Check sheet for the modelled part. Datum: model origin and axes. Units: mm. A direction names the side the tool comes from. Give positions to 0.01 mm unless a question says otherwise; leave off trailing zeros. Loops run counter-clockwise (first coordinate to the right, second up) from the corner with the lowest first, then second, coordinate; pieces in that order, holes last. Notation, with made-up numbers: M 7.5,-7 L 27.5,-7 A14 cw 27.5,10 Z; hole C 81.25,3.25 d1. An arc over 180 degrees is marked long. Put each result on its own line as item: value. Start each with the question number.
```python
from build123d import *

# Parameters (mm, degrees)
F0_W         = 38
F0_H         = 14
F1_DEPTH     = 15
F2_R         = 4.8895
F3_DEPTH     = 15.001
F4_W         = 30.8590809897
F4_H         = 5.2
F5_DEPTH     = 5
F7_DEPTH     = 15.001
F8_W         = 13.0838444641
F8_H         = 13.9913465828
F9_DEPTH     = 8
F11_R        = 0.75
F12_DEPTH    = 15.001
F13_R        = 0.5
F14_T1_DEPTH = 9.498744071
F14_T3_DEPTH = 10.5
F14_T5_DEPTH = 20


# Not quite as in the source:
# - a fillet or chamfer that OpenCascade refuses, or shapes differently, is made with other operations: its cross-section is extruded or revolved along the edge and cut away or added


with BuildPart() as f1:
    # F0 (on Top) → F1 (new body)
    with BuildSketch(Plane.XY):
        with Locations((19, 7)):
            Rectangle(F0_W, F0_H)
    extrude(amount=F1_DEPTH)

    # F2 (on face) → F3 (cut, through all)
    with BuildSketch(Plane.XY.offset(15)):
        with Locations((3, 7)):
            Circle(F2_R)
    extrude(amount=-F3_DEPTH, mode=Mode.SUBTRACT)

    # F4 (on face) → F5 (cut)
    with BuildSketch(Plane(origin=(0, 0, 0), x_dir=(1, 0, 0), z_dir=(0, 0, -1))):
        with Locations((22.5704595052, -7)):
            Rectangle(F4_W, F4_H)
    extrude(amount=-F5_DEPTH, mode=Mode.SUBTRACT)

    # F6 (on face) → F7 (cut, through all)
    with BuildSketch(Plane.XY.offset(15)):
        with BuildLine():
            ThreePointArc((7.60725, 3.1564017591), (4.0503160688, 1.0926455874), (0, 1.8038475773))
            Line((0, 1.8038475773), (0, 0))
            Line((0, 0), (11.143, 0))
            Line((11.143, 0), (11.1420263596, 1.9376011727))
            ThreePointArc((11.1420263596, 1.9376011727), (9.7949393865, 3.7659627841), (7.60725, 3.1564017591))
        make_face()
        with BuildLine():
            ThreePointArc((0, 12.1961524227), (4.0503160688, 12.9073544126), (7.60725, 10.8435982409))
            ThreePointArc((7.60725, 10.8435982409), (9.7949393865, 10.2340372159), (11.1420263596, 12.0623988273))
            Line((11.1420263596, 12.0623988273), (11.1420263596, 14))
            Line((11.1420263596, 14), (0, 14))
            Line((0, 14), (0, 12.1961524227))
        make_face()
    extrude(amount=-F7_DEPTH, mode=Mode.SUBTRACT)

    # F8 (on face) → F9 (cut)
    with BuildSketch(Plane(origin=(0, 0, 0), x_dir=(1, 0, 0), z_dir=(0, 0, -1))):
        with Locations((4.6010777679, -6.9956732914)):
            Rectangle(F8_W, F8_H)
    extrude(amount=-F9_DEPTH, mode=Mode.SUBTRACT)

    # F11 (on face) → F12 (cut, through all)
    with BuildSketch(Plane.XY.offset(15)):
        with Locations((35, 7)):
            Circle(F11_R)
    extrude(amount=-F12_DEPTH, mode=Mode.SUBTRACT)

    # F13
    f13_edges = [f1.edges().sort_by_distance(p)[0] for p in [
        (0, 10.860986, 11.5),
        (0, 3.139014, 11.5),
    ]]
    fillet(f13_edges, radius=F13_R)

    # F14: fillet of radius 1 on 5 edges, made by hand

    # F14_s2 → F14_t1 (cut)
    with BuildSketch(Plane.XY.offset(8)):
        with BuildLine():
            ThreePointArc((11.1424977547, 0.9994975022), (11.4355685293, 0.2927155813), (12.1424976284, 0))
            Line((12.1424976284, 0), (11.143, 0))
            Line((11.143, 0), (11.1424977547, 0.9994975022))
        make_face()
    extrude(amount=F14_T1_DEPTH, mode=Mode.SUBTRACT)

    # F14_s4 → F14_t3 (cut)
    with BuildSketch(Plane.XY.offset(-2.5)):
        with BuildLine():
            ThreePointArc((11.143, 1), (11.4358932188, 0.2928932188), (12.143, 0))
            Line((12.143, 0), (11.143, 0))
            Line((11.143, 0), (11.143, 1))
        make_face()
    extrude(amount=F14_T3_DEPTH, mode=Mode.SUBTRACT)

    # F14_s6 → F14_t5 (cut)
    with BuildSketch(Plane.XY.offset(-2.5)):
        with BuildLine():
            ThreePointArc((37, 0), (37.7071067812, 0.2928932188), (38, 1))
            Line((38, 1), (38, 0))
            Line((38, 0), (37, 0))
        make_face()
        with BuildLine():
            ThreePointArc((11.1420263596, 13), (11.4349195784, 13.7071067812), (12.1420263596, 14))
            Line((12.1420263596, 14), (11.1420263596, 14))
            Line((11.1420263596, 14), (11.1420263596, 13))
        make_face()
        with BuildLine():
            ThreePointArc((38, 13), (37.7071067812, 13.7071067812), (37, 14))
            Line((37, 14), (38, 14))
            Line((38, 14), (38, 13))
        make_face()
    extrude(amount=F14_T5_DEPTH, mode=Mode.SUBTRACT)


solid = f1.part
```
Q1. Section check C-C, the plane x = 3. Record the cut outline in (y, z), then the cut area to 3 significant figures.
Q2. Thickness scan on line 1 along Y through (x, z) = (35, 8); line 2 along Y through (x, z) = (3, 13); line 3 along X through (y, z) = (10.75, 0.75). Record the ranges inside material, lowest first. Write a range as [from, to].
Q3. Section check B-B, the plane x = 35. Record the cut outline in (y, z).
Q4. Section check D-D, the plane z = 9.75. Record the cut outline in (x, y).
Q5. Access from +Z, -Z, +X, -X, +Y, -Y to the whole of each face (thin tool, end or side, straight path). Record for faces 1 (the face through (3.992, 12.917, 11.549)), 2 (the face through (11.143, 7, 6)), 3 (the face through (24, 4.4, 2)).
Q6. Section check A-A, the plane z = 1.5. Record the cut outline in (x, y).
Q7. Depth check by flat-ended pin: P1, Ø1, axis at y = 8.5, z = 13.5, coming from the -X side; P2, Ø6.5, axis at y = 7, z = 3, coming from the -X side; P3, Ø2, axis at x = 7.5, y = 9.5, coming from the -Z side. Enter the tip coordinate at first touch or a pass-through.
Q8. Mould release check, pull along Y, two halves, no side actions. Record for faces 4 (the face through (9.827, 3.755, 11.549)), 5 (the face through (35.715, 7.225, 10.07)), 6 (the face through (9.763, 10.223, 11.549)): pulls with the +Y half, pulls with the -Y half, needs draft (parallel to the pull), parting line crosses it, or undercut.
Found:
1. outline: M 1,8 L 2.11,8 L 2.11,15 L 1,15 Z; M 11.89,8 L 13,8 L 13,15 L 11.89,15 Z
1. area: 15.5 mm^2
2. line 1: y = [0, 6.25], [7.75, 14]
2. line 2: y = [1, 2.11], [11.89, 13]
2. line 3: x = [11.14, 38]
3. outline: M 0,0 L 4.4,0 L 4.4,5 L 6.25,5 L 6.25,15 L 0,15 Z; M 7.75,5 L 9.6,5 L 9.6,0 L 14,0 L 14,15 L 7.75,15 Z
4. outline: M 0,1.8 A6 ccw 7.61,3.16 A2 cw 11.14,1.94 L 11.14,1 A1 ccw 12.14,0 L 37,0 A1 ccw 38,1 L 38,13 A1 ccw 37,14 L 12.14,14 A1 ccw 11.14,13 L 11.14,12.06 A2 cw 7.61,10.84 A6 ccw 0,12.2 L 0,11.77 A0.5 ccw 0.73,11.33 A4.89 cw long 0.73,2.67 A0.5 ccw 0,2.23 Z; hole C 35,7 d1.5
5. face 1: +Z, -Z, +Y
5. face 2: -Z, -X, +Y, -Y
5. face 3: -Z, +X, -X
6. outline: M 11.14,1 A1 ccw 12.14,0 L 37,0 A1 ccw 38,1 L 38,4.4 L 11.14,4.4 Z; M 11.14,9.6 L 38,9.6 L 38,13 A1 ccw 37,14 L 12.14,14 A1 ccw 11.14,13.04 Z
7. P1: stops at x = 7.46
7. P2: stops at x = 11.14
7. P3: stops at z = 8
8. face 4: pulls with the -Y half
8. face 5: undercut
8. face 6: pulls with the +Y half
